Geometry check sheet. Reference: drawing and pictorial views, mm from the part's lowest x, y, z. Round coordinates to 2 decimals unless told otherwise and drop trailing zeros. Order: outer loops, then holes, each group sorted by start corner. A loop starts at its lowest first (then second) coordinate and runs counter-clockwise, first axis right, second up.
(1) Sectioned sample at A-A (z = 25). Record the boundary of the cut face in (x, y).
(2) Release check for a two-part mould opening along Y. For the marked faces 1, 2, 3 and 4 record: +Y half, -Y half, draft (parallel to the pull), parting line (faces both ways), or undercut.
(3) Sectioned sample at B-B (y = 31). Record the boundary of the cut face in (x, z).
(4) Sectioned sample at C-C (x = 15). Record the boundary of the cut face in (y, z).
(5) Go/stop test with flat-tipped pins: pin 1 (10 mm diameter, centred on x = 24.5, z = 10.5, fed in from -Y); pin 2 (5 mm diameter, centred on y = 30.5, z = 32.5, fed in from -X); pin 3 (4 mm diameter, centred on x = 11, z = 21.5, fed in from +Y); pin 4 (18 mm diameter, centred on y = 25, z = 25, fed in from -X). Record where each tip stops, or that it passes through.
(6) Material ranges on line 1 along Z through (x, y) = (14.8, 3.1); line 2 along Y through (x, z) = (46.2, 25); line 3 along Y through (x, z) = (18.5, 37.5), recorded low to high.
(7) Sectioned sample at D-D (z = 40). Record the boundary of the cut face in (x, y), plus the area to 3 significant figures.
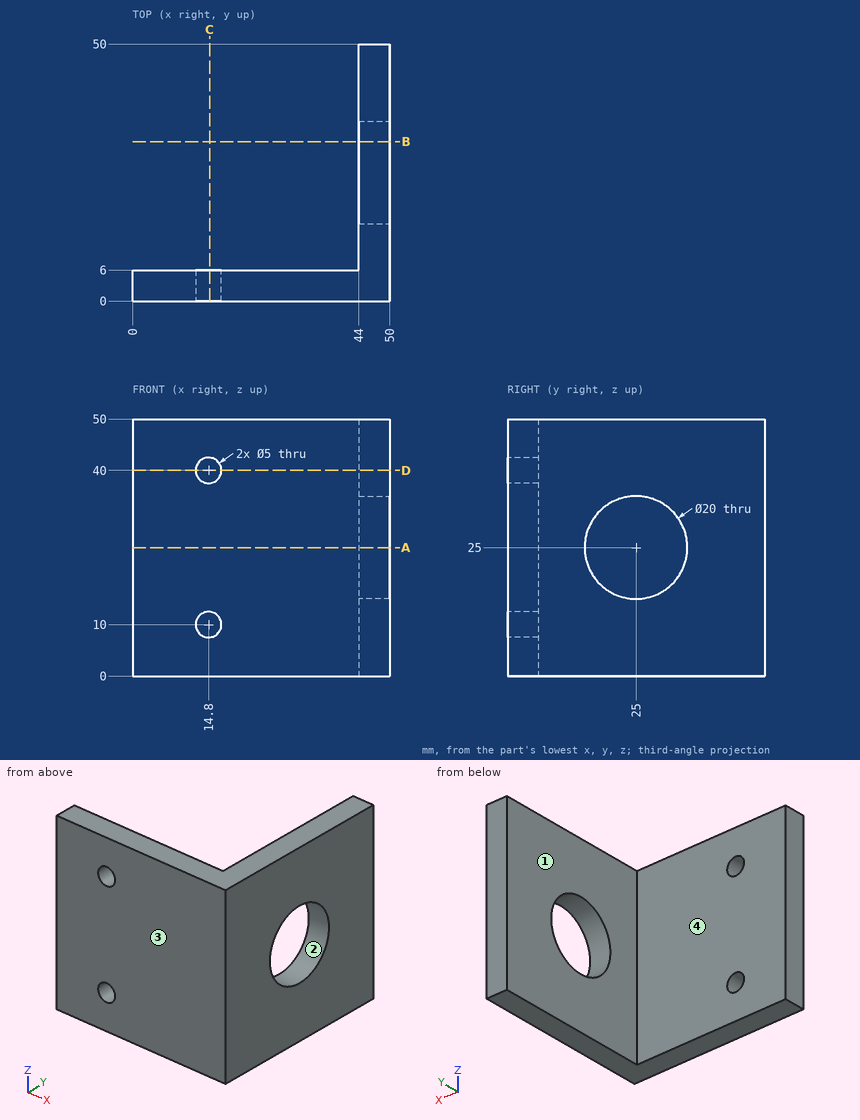
Answer below:
1. outline: (0, 0) - (50, 0) - (50, 15) - (44, 15) - (44, 6) - (0, 6) - close; (44, 35) - (50, 35) - (50, 50) - (44, 50) - close
2. face 1: draft
2. face 2: undercut
2. face 3: -Y half
2. face 4: +Y half
3. outline: (44, 0) - (50, 0) - (50, 17) - (44, 17) - close; (44, 33) - (50, 33) - (50, 50) - (44, 50) - close
4. outline: (0, 0) - (6, 0) - (6, 7.51) - (0, 7.51) - close; (0, 12.49) - (6, 12.49) - (6, 37.51) - (0, 37.51) - close; (0, 42.49) - (6, 42.49) - (6, 50) - (0, 50) - close
5. pin 1: stops at y = 0
5. pin 2: stops at x = 44
5. pin 3: stops at y = 6
5. pin 4: passes through
6. line 1: z = 0 to 7.5, 12.5 to 37.5, 42.5 to 50
6. line 2: y = 0 to 15, 35 to 50
6. line 3: y = 0 to 6
7. outline: (0, 0) - (12.3, 0) - (12.3, 6) - (0, 6) - close; (17.3, 0) - (50, 0) - (50, 50) - (44, 50) - (44, 6) - (17.3, 6) - close
7. area: 534 mm2
